Autodesk Inventor part; units mm, degrees
ref_plane "YZ Plane" through (0, 0, 0) normal (1, 0, 0) x (0, 1, 0)
ref_plane "XZ Plane" through (0, 0, 0) normal (0, 1, 0) x (-1, 0, 0)
ref_plane "XY Plane" through (0, 0, 0) normal (0, 0, 1) x (1, 0, 0)
sketch "Sketch1" plane through (0, 0, 0) normal (0, 1, 0) x (-1, 0, 0)
  circle A0 centre (0, 0) radius 110.292
  dimension "d0" = 220.584
extrude "Extrusion1" add sketch "Sketch1" along normal blind 2
sketch "Sketch2" plane through (0, 2, 0) normal (0, 1, 0) x (1, 0, 0)
  line L0 (0, 0) -> (0, 101.796)
  circle A0 centre (0, 101.796) radius 2
  circle A1 centre (-31.4567, 96.8137) radius 2
  circle A2 centre (-59.8342, 82.3547) radius 2
  circle A3 centre (-82.3547, 59.8342) radius 2
  circle A4 centre (-96.8137, 31.4567) radius 2
  circle A5 centre (-101.796, 0) radius 2
  circle A6 centre (-96.8137, -31.4567) radius 2
  circle A7 centre (-82.3547, -59.8342) radius 2
  circle A8 centre (-59.8342, -82.3547) radius 2
  circle A9 centre (-31.4567, -96.8137) radius 2
  circle A10 centre (0, -101.796) radius 2
  circle A11 centre (31.4567, -96.8137) radius 2
  circle A12 centre (59.8342, -82.3547) radius 2
  circle A13 centre (82.3547, -59.8342) radius 2
  circle A14 centre (96.8137, -31.4567) radius 2
  circle A15 centre (101.796, 0) radius 2
  circle A16 centre (96.8137, 31.4567) radius 2
  circle A17 centre (82.3547, 59.8342) radius 2
  circle A18 centre (59.8342, 82.3547) radius 2
  circle A19 centre (31.4567, 96.8137) radius 2
  dimension "d3" = 101.796
  dimension "d4" = 4
  dimension "d7" = 360
hole "Hole1" at (-96.8137, 2, -31.4567) at (-82.3547, 2, -59.8342) at (-59.8342, 2, -82.3547) at (-31.4567, 2, -96.8137) at (31.4567, 2, -96.8137) at (59.8342, 2, -82.3547) at (82.3547, 2, -59.8342) at (96.8137, 2, -31.4567) at (101.796, 2, 0) at (96.8137, 2, 31.4567) at (82.3547, 2, 59.8342) at (59.8342, 2, 82.3547) at (31.4567, 2, 96.8137) at (0, 2, 101.796) at (-31.4567, 2, 96.8137) at (-59.8342, 2, 82.3547) at (-82.3547, 2, 59.8342) at (-96.8137, 2, 31.4567) at (-101.796, 2, 0) at (0, 2, -101.796) direction (0, -1, 0) diameter 4 end through all
sketch "Sketch4" plane through (0, 2, 0) normal (0, 1, 0) x (1, 0, 0)
  point P0 (0, 0)
  point P1 (0, 0)
hole "Hole2" at (0, 2, 0) direction (0, -1, 0) diameter 6 end through all
properties part number "baseplate_azimuth_gear" material "Aluminum 6061"
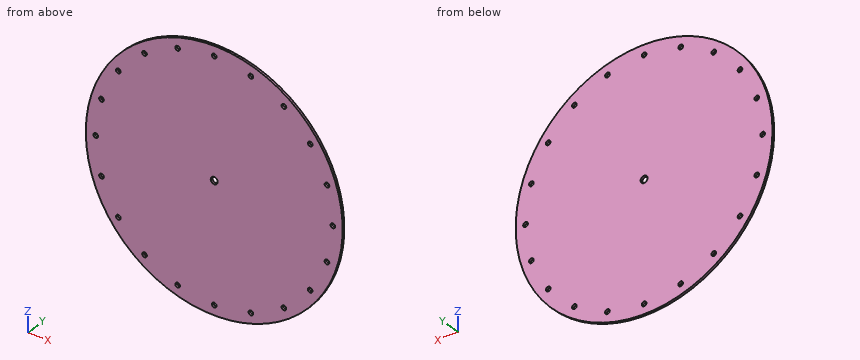
Build history of the part. All positions in model axes, mm. Give positions to 0.01 mm unless a question says otherwise; leave off trailing zeros. Order: outer loops, then holes, each group sorted by start corner. A loop starts at its lowest first (then second) coordinate and runs counter-clockwise, first axis right, second up. Notation, with made-up numbers: M -20.5,79.25 L 36.5,79.25 A6 ccw 36.5,89.25 Z; hole C 77,-33.5 d1. An arc over 180 degrees is marked long. Put each result on its own line as item: value.
Item 1: Probe line 1 (Z direction, x = 0, y = 0.5); line 2 (X direction, y = 1.8, z = -97); line 3 (Z direction, x = 96, y = 0.6). List the from-to ranges inside material, lowest first. Write a range as [from, to].
From the geometry:
line 1: z = [-110.29, -103.8], [-99.8, -3], [3, 99.8], [103.8, 110.29]
line 2: x = [-52.49, -33.45], [-29.47, 29.47], [33.45, 52.49]
line 3: z = [-54.3, -33.28], [-29.63, 29.63], [33.28, 54.3]
Item 2: Slice it at C-C, the plane x = 72.5. Write the cut outline in (y, z), plus the area to 3 significant figures.
From the geometry:
outline: M 0,-83.11 L 2,-83.11 L 2,83.11 L 0,83.11 Z
area: 332 mm2
Item 3: Slice it at A-A, the plane y = 0.85. Give the number of separate pieces and of enclosed holes in the cut face, plus the area to 3 significant figures.
From the geometry:
separate pieces: 1
enclosed holes: 21
area: 37,900 mm2
Item 4: Slice it at B-B, the plane z = -75. Write the cut outline in (x, y), plus the area to 3 significant figures.
From the geometry:
outline: M -80.87,0 L 80.87,0 L 80.87,2 L -80.87,2 Z
area: 323 mm2
Item 5: Flat gauge pins, fed straight in: pin 1 Ø6.5 at (x, z) = (82.35, -59.83) entering from -Y; pin 2 Ø1 at (x, y) = (66, 1) entering from -Z; pin 3 Ø2.5 at (x, z) = (-31.46, 96.81) entering from +Y. Where does each tip first touch, or does it go through?
From the geometry:
pin 1: stops at y = 0
pin 2: stops at z = -88.74
pin 3: passes through
